Verification items for the finished model (mm, model axes). A direction names the side the tool comes from. Coordinates: 2 decimals unless noted, no trailing zeros. Write each loop counter-clockwise with the first axis right and the second up, starting at its lowest first coordinate (ties: lowest second). Pieces come first, ordered by that corner, then holes. Notation, with made-up numbers: M 88,-5 L 143,-5 A16 cw 143,14 Z; hole C 34,-1 d4. An arc over 180 degrees is marked long. Answer in a Markdown table with one row per item.
from build123d import *

# Parameters (mm, degrees)
F0_R      = 2.5
F1_DEPTH  = 6
F5_DEPTH  = 0.7
F6_W      = 0.6
F6_H      = 0.6
F7_DEPTH  = 2
F7_FACE_W = 0.6
F7_FACE_H = 0.6
F8_DEPTH  = 1


with BuildPart() as f1:
    # F0 (on Top) → F1 (new body)
    with BuildSketch(Plane.XY):
        Circle(F0_R)
    extrude(amount=F1_DEPTH)

    # F2 (on face) → F3 (revolve)
    with BuildSketch(Plane.XY.offset(6)):
        with BuildLine():
            ThreePointArc((0, 2.5), (-2.5, 0), (0, -2.5))
            Line((0, -2.5), (0, 2.5))
        make_face()
    revolve(axis=Axis((0, 0, 6), (0, 1, 0)))

    # F4 (on face) → F5 (join)
    with BuildSketch(Plane(origin=(0, 0, 0), x_dir=(1, 0, 0), z_dir=(0, 0, -1))):
        with BuildLine():
            Line((-2.5, 1.658312), (-2.5, -1.658312))
            ThreePointArc((-2.5, -1.658312), (3, 0), (-2.5, 1.658312))
        make_face()
    extrude(amount=-F5_DEPTH)

    # F6 (on face) → F7 (join)
    with BuildSketch(Plane(origin=(0, 0, 0), x_dir=(1, 0, 0), z_dir=(0, 0, -1))):
        with Locations((1.25, 0)):
            Rectangle(F6_W, F6_H)
        with Locations((-1.25, 0)):
            Rectangle(F6_W, F6_H)
    extrude(amount=F7_DEPTH)

    # F7_face (on face) → F8 (join)
    with BuildSketch(Plane(origin=(1.25, 0, -2), x_dir=(1, 0, 0), z_dir=(0, 0, -1))):
        Rectangle(F7_FACE_W, F7_FACE_H)
    extrude(amount=F8_DEPTH)


solid = f1.part
1) Sectioned sample at C-C (y = -2.25). Record the cut outline in (x, z), then the cut area to 3 significant figures.
Response values:
| item | result |
|---|---|
| outline | M -1.98,0 L 1.98,0 L 1.98,0.7 L 1.09,0.7 L 1.09,6 A1.09 ccw -1.09,6 L -1.09,0.7 L -1.98,0.7 Z |
| area | 16.2 mm² |
2) Sectioned sample at D-D (z = 4.75). Record the cut outline in (x, y), then the cut area to 3 significant figures.
Response values:
| item | result |
|---|---|
| outline | C 0,0 d5 |
| area | 19.6 mm² |
3) Sectioned sample at A-A (z = -0.25). Record the cut outline in (x, y), then the cut area to 3 significant figures.
Response values:
| item | result |
|---|---|
| outline | M -1.55,-0.3 L -0.95,-0.3 L -0.95,0.3 L -1.55,0.3 Z; M 0.95,-0.3 L 1.55,-0.3 L 1.55,0.3 L 0.95,0.3 Z |
| area | 0.720 mm² |
4) Depth check by flat-ended pin: pin 1 (0.7 mm diameter, centred on x = 1.5, z = -1.5, fed in from +Y); pin 2 (0.7 mm diameter, centred on x = -1.5, y = 0, fed in from -Z); pin 3 (0.5 mm diameter, centred on x = -1, z = -1, fed in from -Y). Enter the tip coordinate at first touch or a pass-through.
Response values:
| item | result |
|---|---|
| pin 1 | stops at y = 0.3 |
| pin 2 | stops at z = -2 |
| pin 3 | stops at y = -0.3 |
5) Thickness scan on L1, parallel to X at y = 0.1, z = 5.5; L2, parallel to X at y = -2.1, z = 5; L3, parallel to Y at x = 1.65, z = 3.25. Record the ranges inside material, lowest first. Write a range as [from, to].
Response values:
| item | result |
|---|---|
| L1 | x = [-2.5, 2.5] |
| L2 | x = [-1.36, 1.36] |
| L3 | y = [-1.88, 1.88] |
6) Sectioned sample at B-B (x = 0). Record the cut outline in (y, z).
Response values:
| item | result |
|---|---|
| outline | M -3,0 L 3,0 L 3,0.7 L 2.5,0.7 L 2.5,6 A2.5 ccw -2.5,6 L -2.5,0.7 L -3,0.7 Z |
7) Tool access check on faces 1 (the face through (-0.54, -2.44, 3.31)), 2 (the face through (3, 0.1, 0.3)). Record the directions out of +Z, -Z, +X, -X, +Y, -Y that give a thin tool (end or side, any length) a straight path to the whole face; none if there is none.
Response values:
| item | result |
|---|---|
| face 1 | +Z |
| face 2 | +Z, -Z |
